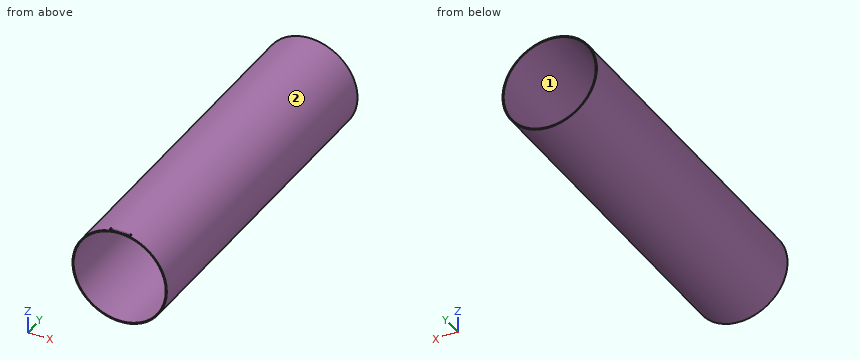
from build123d import *

# Parameters (mm, degrees)
SKETCH1_R           = 52.07
SKETCH1_R_2         = 50.8
BOSS_EXTRUDE1_DEPTH = 381
BOSS_EXTRUDE2_DEPTH = 2.54


with BuildPart() as part:
    # Sketch1 → Boss-Extrude1 (new body)
    with BuildSketch(Plane(origin=(0, 0, 0), x_dir=(1, 0, 0), z_dir=(0, 1, 0))):
        Circle(SKETCH1_R)
        Circle(SKETCH1_R_2, mode=Mode.SUBTRACT)
    extrude(amount=BOSS_EXTRUDE1_DEPTH)

    # Sketch2 → Boss-Extrude2 (add)
    with BuildSketch(Plane.XZ):
        with BuildLine():
            ThreePointArc((-11.43, 50.8), (-5.750169563, 51.751526064), (0, 52.07))
            Line((0, 52.07), (-11.43, 52.07))
            Line((-11.43, 52.07), (-11.43, 50.8))
        make_face()
        with BuildLine():
            Line((11.43, 52.07), (0, 52.07))
            ThreePointArc((0, 52.07), (5.750169563, 51.751526064), (11.43, 50.8))
            Line((11.43, 50.8), (11.43, 52.07))
        make_face()
    extrude(amount=-BOSS_EXTRUDE2_DEPTH)


solid = part.part
Source: CAD feature listing. Evaluate the final solid. Frame: model axes, mm. Face numbers are marked on the shaded views. Round coordinates to 2 decimals unless told otherwise and drop trailing zeros. Loops run counter-clockwise (first coordinate to the right, second up) from the corner with the lowest first, then second, coordinate; pieces in that order, holes last. Notation, with made-up numbers: (34, 31.25) - (77, 31.25) arc R12 ccw to (77, 51.25) - close; hole circle Ø3 at (44.5, 21.5). An arc over 180 degrees is marked (long way). Write item = value, one per line. Start each with the question number.
(1) Pull-direction query (X, two-part tool) for the marked faces 1 and 2; classes: +X half, -X half, draft (parallel to the pull), parting line (faces both ways), or undercut.
(2) Pin query (flat end, axial travel): pin 1 (5 mm diameter, centred on x = 13, y = 324.5, fed in from +Z); pin 2 (4 mm diameter, centred on x = 18.5, y = 251, fed in from -Z); pin 3 (3 mm diameter, centred on x = -16.5, y = 158, fed in from -Z); pin 4 (12 mm diameter, centred on x = 40.5, z = -5, fed in from +Y). Return the tip coordinate at first contact, or that it passes through.
(3) Ray query, line 1 along X through (y, z) = (113.5, 0); line 2 along Z through (x, y) = (6, 158). Return the intervals inside material, ascending. Write a range as from..to.
(4) Section query A-A, the plane z = 13. Output: boundary loops of the cut face in (x, y), plus the area to 3 significant figures.
(5) Section query C-C, the plane y = 322.5. Output: boundary loops of the cut face in (x, z).
(6) Section query B-B, the plane x = 26. Output: boundary loops of the cut face in (y, z).
Conclusion:
q1.face_1 = undercut
q1.face_2 = parting line
q2.pin_1 = 51
q2.pin_2 = -49.39
q2.pin_3 = -49.86
q2.pin_4 = through
q3.line_1 = -52.07..-50.8, 50.8..52.07
q3.line_2 = -51.72..-50.44, 50.44..51.72
q4.outline = (-50.42, 0) - (-49.11, 0) - (-49.11, 381) - (-50.42, 381) - close; (49.11, 0) - (50.42, 0) - (50.42, 381) - (49.11, 381) - close
q4.area = 1,000 mm2
q5.outline = circle Ø104.14 at (0, 0); hole circle Ø101.6 at (0, 0)
q6.outline = (0, -45.11) - (381, -45.11) - (381, -43.64) - (0, -43.64) - close; (0, 43.64) - (381, 43.64) - (381, 45.11) - (0, 45.11) - close
